Input: part model. Units: mm. Frame: model coordinates. Face numbers are marked on the shaded views. A direction names the side the tool comes from. Give positions to 0.01 mm unless a question says otherwise; leave off trailing zeros. Loops run counter-clockwise (first coordinate to the right, second up) from the corner with the lowest first, then second, coordinate; pieces in that order, holes last.
from build123d import *

# Parameters (mm, degrees)
SKETCH1_R                = 12.7
BOSS_EXTRUDE3_DEPTH      = 152.4
SKETCH9_R                = 6.35
BOSS_EXTRUDE6_DEPTH      = 19.05
SKETCH16_W               = 25.4
SKETCH16_H               = 63.5
CUT_EXTRUDE2_DEPTH       = 155.762931731
SKETCH17_W               = 25.4
SKETCH17_H               = 63.5
CUT_EXTRUDE3_DEPTH       = 155.762931731
SKETCH19_R               = 2.54
CUT_EXTRUDE5_DEPTH       = 155.762931731
SKETCH21_W               = 21.59
SKETCH21_H               = 12.7
BOSS_EXTRUDE8_DEPTH      = 12.7
BOSS_EXTRUDE9_DEPTH      = 6.35
SKETCH25_R               = 3.175
CUT_EXTRUDE7_DEPTH       = 21.59
SKETCH29_R               = 2.921
BOSS_EXTRUDE10_DEPTH     = 35.814
FILLET2_R                = 6.35
FILLET3_R                = 6.35
SKETCH31_W               = 63.5
SKETCH31_H               = 63.5
BOSS_EXTRUDE11_DEPTH     = 10.16
SKETCH32_W               = 76.52614712
SKETCH32_H               = 17.415789338
CUT_EXTRUDE8_DEPTH       = 195.047688304
SKETCH33_W               = 10.16
SKETCH33_H               = 12.7
CUT_EXTRUDE9_DEPTH       = 168.793532357
CUT_EXTRUDE11_DEPTH      = 169.255829122
CUT_EXTRUDE11_DEPTH_BACK = 169.255829122
SKETCH35_R               = 2.921


with BuildPart() as part:
    # Sketch1 → Boss-Extrude3 (new, symmetric)
    with BuildSketch(Plane.XY):
        with Locations(Location((0, 0, 0), (0, 0, 180))):
            Circle(SKETCH1_R)
    extrude(amount=BOSS_EXTRUDE3_DEPTH, both=True)

    # Sketch9 → Boss-Extrude6 (add, symmetric)
    with BuildSketch(Plane(origin=(0, 0, 0), x_dir=(0, 0, -1), z_dir=(1, 0, 0))):
        with Locations((-25.4, 0)):
            Circle(SKETCH9_R)
    extrude(amount=BOSS_EXTRUDE6_DEPTH, both=True)

    # Sketch16 → Cut-Extrude2 (cut, through all)
    with BuildSketch(Plane(origin=(0, -6.35, 0), x_dir=(1, 0, 0), z_dir=(0, 1, 0))):
        with Locations((0, 120.65)):
            Rectangle(SKETCH16_W, SKETCH16_H)
    extrude(amount=-CUT_EXTRUDE2_DEPTH, mode=Mode.SUBTRACT)

    # Sketch17 → Cut-Extrude3 (cut, through all)
    with BuildSketch(Plane(origin=(0, 6.35, 0), x_dir=(1, 0, 0), z_dir=(0, 1, 0))):
        with Locations((0, 120.65)):
            Rectangle(SKETCH17_W, SKETCH17_H)
    extrude(amount=CUT_EXTRUDE3_DEPTH, mode=Mode.SUBTRACT)

    # Sketch19 → Cut-Extrude5 (cut, through all)
    with BuildSketch(Plane(origin=(0, 6.35, 0), x_dir=(1, 0, 0), z_dir=(0, 1, 0))):
        with Locations(Location((0, 100.80625, 0), (0, 0, 270))):
            Circle(SKETCH19_R)
        with Locations(Location((0, 136.525, 0), (0, 0, 270))):
            Circle(SKETCH19_R)
    extrude(amount=-CUT_EXTRUDE5_DEPTH, mode=Mode.SUBTRACT)

    # Sketch21 → Boss-Extrude8 (add)
    with BuildSketch(Plane.XY.offset(152.4)):
        Rectangle(SKETCH21_W, SKETCH21_H)
    extrude(amount=BOSS_EXTRUDE8_DEPTH)

    # Sketch25 → Cut-Extrude7 (cut)
    with BuildSketch(Plane.ZY.offset(10.795)):
        with Locations(Location((158.75, 0, 0), (0, 0, 270))):
            Circle(SKETCH25_R)
    extrude(amount=-CUT_EXTRUDE7_DEPTH, mode=Mode.SUBTRACT)

    # Fillet3
    fillet3_edges = [part.edges().sort_by_distance(p)[0] for p in [
        (0, -6.35, 165.1),
        (0, 6.35, 165.1),
    ]]
    fillet(fillet3_edges, radius=FILLET3_R - 0.0001)  # a hair under: the kernel refuses the full size


with BuildPart() as body_2:
    # Sketch27 → Boss-Extrude9 (new, symmetric)
    with BuildSketch(Plane(origin=(0, 0, 0), x_dir=(1, 0, 0), z_dir=(0, 1, 0))):
        Polygon((0, -165.354), (11.049, -165.354), (11.049, -152.654), (21.209, -152.654), (21.209, -170.434), (-21.209, -170.434), (-21.209, -152.654), (-11.049, -152.654), (-11.049, -165.354), align=None)
    extrude(amount=BOSS_EXTRUDE9_DEPTH, both=True)

    # Sketch29 → Boss-Extrude10 (add)
    with BuildSketch(Plane.ZY.offset(21.209)):
        with Locations((158.827896988, 0)):
            Circle(SKETCH29_R)
    extrude(amount=-BOSS_EXTRUDE10_DEPTH)

    # Fillet2
    fillet2_edges = [body_2.edges().sort_by_distance(p)[0] for p in [
        (16.129, -6.35, 152.654),
        (16.129, 6.35, 152.654),
        (-16.129, -6.35, 152.654),
        (-16.129, 6.35, 152.654),
    ]]
    fillet(fillet2_edges, radius=FILLET2_R - 0.0001)  # a hair under: the kernel refuses the full size

    # Sketch31 → Boss-Extrude11 (add)
    with BuildSketch(Plane.XY.offset(170.434)):
        Rectangle(SKETCH31_W, SKETCH31_H)
    extrude(amount=BOSS_EXTRUDE11_DEPTH)

    # Sketch32 → Cut-Extrude8 (cut, through all)
    with BuildSketch(Plane(origin=(0, 31.75, 0), x_dir=(1, 0, 0), z_dir=(0, 1, 0))):
        with Locations((-0.932221908, -174.061894669)):
            Rectangle(SKETCH32_W, SKETCH32_H)
    extrude(amount=-CUT_EXTRUDE8_DEPTH, mode=Mode.SUBTRACT)

    # Sketch33 → Cut-Extrude9 (cut, through all)
    with BuildSketch(Plane(origin=(0, 6.35, 0), x_dir=(1, 0, 0), z_dir=(0, 1, 0))):
        with Locations((-16.129, -159.004)):
            Rectangle(SKETCH33_W, SKETCH33_H)
        with Locations((16.129, -159.004)):
            Rectangle(SKETCH33_W, SKETCH33_H)
    extrude(amount=-CUT_EXTRUDE9_DEPTH, mode=Mode.SUBTRACT)

    # Sketch35 → Cut-Extrude11 (cut, two sides: drawn at the far end of the back side and taken through both)
    with BuildSketch(Plane.ZY.offset(10.795).offset(-CUT_EXTRUDE11_DEPTH_BACK)):
        with Locations((158.827896988, 0)):
            Circle(SKETCH35_R)
    extrude(amount=CUT_EXTRUDE11_DEPTH + CUT_EXTRUDE11_DEPTH_BACK, mode=Mode.SUBTRACT)


solid = part.part
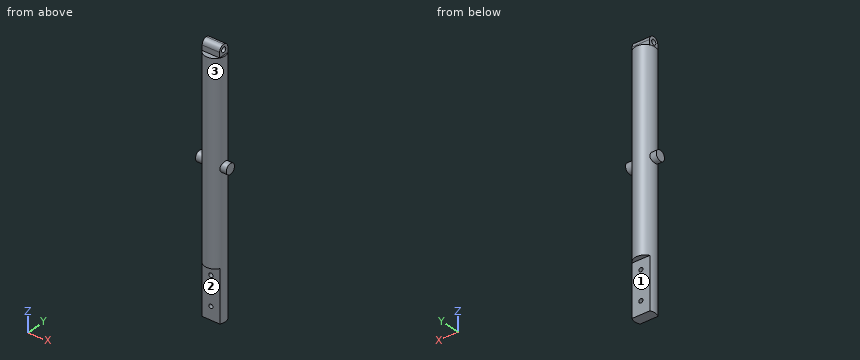
(1) Ray query, probe 1 along Z at (x, y) = (-3.25, 0) (3 decimals); probe 2 along Z at (x, y) = (14, -0.75); probe 3 along X at (y, z) = (1, 52). Return the intervals inside material, ascending.
Values follow:
probe 1: z = -152.4 to 155.575, 161.925 to 165.1
probe 2: z = 19.09 to 31.71
probe 3: x = -12.66 to 12.66
(2) Reachability of the marked faces 1, 2 and 3 from +Z, -Z, +X, -X, +Y, -Y: full face, straight path, thin tool, end or side. Return the list, or none.
Values follow:
face 1: -Z, +X, -X, +Y
face 2: -Z, +X, -X, -Y
face 3: none
(3) Pin query (flat end, axial travel): pin 1 Ø4 at (x, z) = (0, -100.81) entering from +Y; pin 2 Ø7 at (x, y) = (2.5, 11) entering from -Z; pin 3 Ø2 at (x, y) = (-5, 0.5) entering from +Z; pin 4 Ø8 at (x, y) = (10, -9.5) entering from +Z. Return the tip coordinate at first contact, or that it passes through.
Values follow:
pin 1: passes through
pin 2: stops at z = -88.9
pin 3: stops at z = 165.1
pin 4: stops at z = 161.92
(4) Cut plane A-A (z = 25.4). Return the cut outline in (x, y), and give its area (3 significant figures).
Values follow:
outline: (-19.05, -6.35) - (-11, -6.35) arc R12.7 ccw to (11, -6.35) - (19.05, -6.35) - (19.05, 6.35) - (11, 6.35) arc R12.7 ccw to (-11, 6.35) - (-19.05, 6.35) - close
area: 682 mm2
